```python
from build123d import *

# Parameters (mm, degrees)
SKETCH1_W               = 115
SKETCH1_H               = 30
BOSS_EXTRUDE1_DEPTH     = 3
SKETCH2_W               = 120
SKETCH2_H               = 35
SKETCH2_W_2             = 115
SKETCH2_H_2             = 30
BOSS_EXTRUDE3_DEPTH     = 6
SKETCH4_R               = 1
CUT_EXTRUDE1_DEPTH      = 4
LPATTERN1_COUNT         = 7
LPATTERN1_PITCH         = 15
SKETCH5_R               = 1.6
BOSS_EXTRUDE4_DEPTH     = 3
MIRROR2_COPY_1_SKETCH_R = 1.6
MIRROR2_COPY_1_DEPTH    = 3


with BuildPart() as part:
    # Sketch1 → Boss-Extrude1 (new body)
    with BuildSketch(Plane(origin=(0, 0, 0), x_dir=(1, 0, 0), z_dir=(0, 1, 0))):
        with Locations((57.5, 15)):
            Rectangle(SKETCH1_W, SKETCH1_H)
    extrude(amount=BOSS_EXTRUDE1_DEPTH)

    # Sketch2 → Boss-Extrude3 (add)
    with BuildSketch(Plane(origin=(0, 0, 0), x_dir=(1, 0, 0), z_dir=(0, 1, 0))):
        with Locations((57.5, 15)):
            Rectangle(SKETCH2_W, SKETCH2_H)
        with Locations((57.5, 15)):
            Rectangle(SKETCH2_W_2, SKETCH2_H_2, mode=Mode.SUBTRACT)
    extrude(amount=BOSS_EXTRUDE3_DEPTH)

    # Sketch4 → Cut-Extrude1 (cut, symmetric)
    with BuildSketch(Plane(origin=(0, 3, 0), x_dir=(1, 0, 0), z_dir=(0, 1, 0))):
        with Locations((10, 10)):
            Circle(SKETCH4_R)
    cut_extrude1 = extrude(amount=CUT_EXTRUDE1_DEPTH, both=True, mode=Mode.SUBTRACT)

    # LPattern1: Cut-Extrude1 ×7
    with Locations(*[(i * LPATTERN1_PITCH, 0, 0) for i in range(1, LPATTERN1_COUNT)]):
        add(cut_extrude1, mode=Mode.SUBTRACT)

    # Sketch5 → Boss-Extrude4 (add)
    with BuildSketch(Plane(origin=(0, 0, 0), x_dir=(1, 0, 0), z_dir=(0, 1, 0))):
        with BuildLine():
            Line((-2.5, -2.5), (-2.5, -7.5))
            ThreePointArc((-2.5, -7.5), (1, -11), (4.5, -7.5))
            Line((4.5, -7.5), (4.5, -2.5))
            Line((4.5, -2.5), (-2.5, -2.5))
        make_face()
        with Locations((1, -7.5)):
            Circle(SKETCH5_R, mode=Mode.SUBTRACT)
    boss_extrude4 = extrude(amount=BOSS_EXTRUDE4_DEPTH)

    # Mirror1: Boss-Extrude4 across plane
    add(boss_extrude4.mirror(Plane.XY.offset(-15)))

    # Mirror2: Boss-Extrude4 across plane
    add(boss_extrude4.mirror(Plane.ZY.offset(-57.5)))

    # Mirror2 copy 1 sketch → Mirror2 copy 1 (add)
    with BuildSketch(Plane(origin=(115, 0, -30), x_dir=(-1, 0, 0), z_dir=(0, 1, 0))):
        with BuildLine():
            Line((-2.5, -2.5), (-2.5, -7.5))
            ThreePointArc((-2.5, -7.5), (1, -11), (4.5, -7.5))
            Line((4.5, -7.5), (4.5, -2.5))
            Line((4.5, -2.5), (-2.5, -2.5))
        make_face()
        with Locations((1, -7.5)):
            Circle(MIRROR2_COPY_1_SKETCH_R, mode=Mode.SUBTRACT)
    extrude(amount=MIRROR2_COPY_1_DEPTH)


solid = part.part
```
Geometry check sheet. Reference: the model listing, model coordinates, mm. A direction names the side the tool comes from. Round coordinates to 2 decimals unless told otherwise and drop trailing zeros. Order: outer loops, then holes, each group sorted by start corner. A loop starts at its lowest first (then second) coordinate and runs counter-clockwise, first axis right, second up. Notation, with made-up numbers: (25, 46) - (70, 46) arc R10 cw to (70, 56) - close; hole circle Ø4 at (6, 78). An arc over 180 degrees is marked (long way). Use a Markdown table: item, result. Add a question column.
1) Section check A-A (y = 5.05). Record the cut outline in (x, z).
2) Section check B-B (z = -13.5). Record the cut outline in (x, y).
3) Gauge pin test, flat ends, axial feed: P1, Ø1.5, axis at x = 34.5, z = -14, coming from the +Y side; P2, Ø3.5, axis at x = 77, y = 4.5, coming from the +Z side. Record the tip position at first contact, or that the pin passes through.
4) Set-up check for faces 5 (the flat face through (114, 3, -35.7)), 6 (the flat face through (4.5, 1, 5)), 7 (the flat face through (115, 4, -15)), 8 (the flat face through (1, 3, 5.7)), 9 (the flat face through (4.5, 1, -35)): record each of +Z, -Z, +X, -X, +Y, -Y from which the full face is reachable in a straight line by a thin tool's end or side.
5) Section check C-C (x = 43.5). Record the cut outline in (y, z), then the cut area to 3 significant figures.
6) Thickness scan on line 1 along X through (y, z) = (1.9, 7.5); line 2 along Z through (x, y) = (47.5, 4.35); line 3 along Z through (x, y) = (114, 2.3). Record the ranges inside material, lowest first.
7) Mould release check, pull along X, two halves, no side actions. Record for faces 1 (the flat face through (-2.5, 3, -15)), 2 (the flat face through (57, 4, -30)), 3 (the flat face through (48.3, 6, 0.5)), 4 (the cylindrical face through (114, 1, -41)): released by +X, released by -X, zero draft, split by the parting line, or undercut.
Established:
| question | item | result |
|---|---|---|
| 1 | outline | (-2.5, -32.5) - (117.5, -32.5) - (117.5, 2.5) - (-2.5, 2.5) - close; hole (0, -30) - (115, -30) - (115, 0) - (0, 0) - close |
| 2 | outline | (-2.5, 0) - (117.5, 0) - (117.5, 6) - (115, 6) - (115, 3) - (0, 3) - (0, 6) - (-2.5, 6) - close |
| 3 | P1 | y = 3 |
| 3 | P2 | z = 2.5 |
| 4 | face 5 | -Z, +X, -X, +Y |
| 4 | face 6 | +Z, +Y, -Y |
| 4 | face 7 | +Y |
| 4 | face 8 | +Z, +X, -X, +Y |
| 4 | face 9 | -Z, +Y, -Y |
| 5 | outline | (0, -32.5) - (6, -32.5) - (6, -30) - (3, -30) - (3, 0) - (6, 0) - (6, 2.5) - (0, 2.5) - close |
| 5 | area | 120 mm2 |
| 6 | line 1 | -2.5 to -0.6, 2.6 to 4.5, 110.5 to 112.4, 115.6 to 117.5 |
| 6 | line 2 | -32.5 to -30, 0 to 2.5 |
| 6 | line 3 | -41 to -39.1, -35.9 to 5.9, 9.1 to 11 |
| 7 | face 1 | released by -X |
| 7 | face 2 | undercut |
| 7 | face 3 | zero draft |
| 7 | face 4 | undercut |
